Check sheet for the drawn part. Datum: minimum x, y, z corner. Units: mm. A direction names the side the tool comes from. Round coordinates to 2 decimals unless told otherwise and drop trailing zeros. Order: outer loops, then holes, each group sorted by start corner. A loop starts at its lowest first (then second) coordinate and runs counter-clockwise, first axis right, second up. Notation, with made-up numbers: (45.5, 18) - (91.5, 18) arc R13 ccw to (91.5, 33) - close; hole circle Ø5 at (87.25, 41). An arc over 180 degrees is marked (long way). Write each question's results on one line, items separated by ' | '.
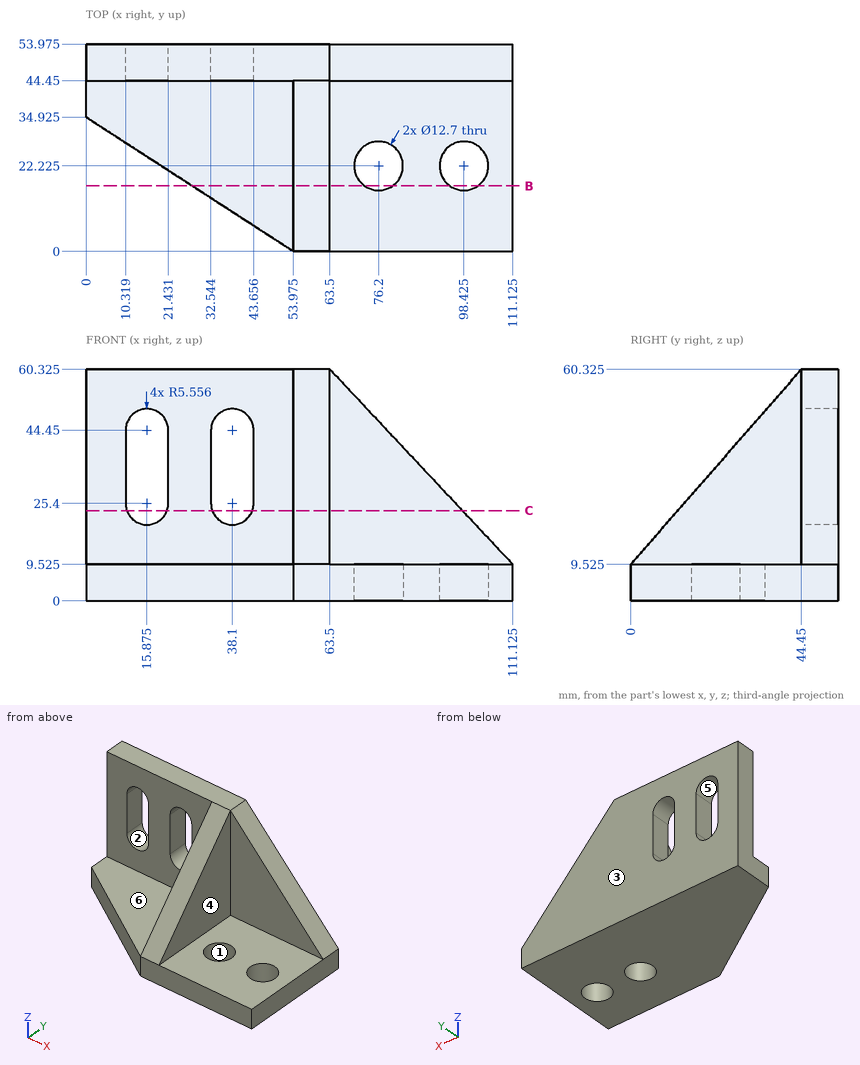
(1) Draft check along Y on the marked faces 1, 2 and 3. Enter one of: released by +Y, released by -Y, zero draft, split by the parting line, or undercut.
Answers follow:
face 1: undercut | face 2: zero draft | face 3: released by +Y
(2) Section check C-C (z = 23.5). Give the number of separate pieces and of enclosed holes in the cut face, then the cut area to 3 significant figures.
Answers follow:
separate pieces: 3 | enclosed holes: 0 | area: 1,040 mm²
(3) Section check B-B (y = 17). Record the cut outline in (x, z) (1 decimal), then the cut area to 3 significant figures.
Answers follow:
outline: (27.7, 0) - (72.6, 0) - (72.6, 9.5) - (63.5, 9.5) - (63.5, 29) - (54, 29) - (54, 9.5) - (27.7, 9.5) - close; (79.8, 0) - (94.8, 0) - (94.8, 9.5) - (79.8, 9.5) - close; (102, 0) - (111.1, 0) - (111.1, 9.5) - (102, 9.5) - close | area: 842 mm²
(4) Material ranges on line 1 (X direction, y = 50, z = 22) (1 decimal); line 2 (X direction, y = 33, z = 12) (1 decimal); line 3 (Z direction, x = 79, y = 36.5) (1 decimal), recorded low to high.
Answers follow:
line 1: 0 to 11.5, 20.3 to 33.7, 42.5 to 99.4 | line 2: 54 to 63.5 | line 3: 0 to 9.5
(5) Depth check by flat-ended pin: pin 1 Ø13.5 at (x, y) = (94, 19.5) entering from +Z (3 decimals); pin 2 Ø3 at (y, z) = (48.5, 38) entering from +X (1 decimal); pin 3 Ø8 at (y, z) = (14.5, 32) entering from -X (3 decimals). Enter the tip coordinate at first touch or a pass-through.
Answers follow:
pin 1: z = 9.525 | pin 2: x = 85.8 | pin 3: x = 53.975
(6) Access from +Z, -Z, +X, -X, +Y, -Y to the whole of each face (thin tool, end or side, straight path). Record for the marked faces 4, 5 and 6.
Answers follow:
face 4: +Z, +X, -Y | face 5: +Y, -Y | face 6: +Z, -X, -Y
